Can you work these out from the model? Positions are in its coordinate system, mm. A direction names the side the tool comes from. Give positions to 0.01 mm unless a question says otherwise; leave off trailing zeros. Write each loop counter-clockwise with the first axis right and the second up, starting at its lowest first coordinate (ties: lowest second). Pieces come first, ordered by that corner, then holes. Notation, with made-up numbers: M -21.5,66 L -6.5,66 A33 cw -6.5,101 Z; hole C -4.5,-24 d9. An arc over 180 degrees is marked long. Write each question's results on one line, items separated by ' | '.
from build123d import *

# Parameters (mm, degrees)
F1_DEPTH = 117.094
F4_DEPTH = 25.4
F2_R     = 16.9643352209
F2_R_2   = 9.9441
F5_DEPTH = 65.278


with BuildPart() as f1:
    # F0 (on Front) → F1 (new body)
    with BuildSketch(Plane.XZ):
        Polygon((-76.2, 0), (0, 0), (0, 152.4), (-30.48, 152.4), (-30.48, 25.4), (-76.2, 25.4), align=None)
    extrude(amount=F1_DEPTH)

    # F3 (on face) → F4 (cut)
    with BuildSketch(Plane.XY.offset(25.4)):
        with BuildLine():
            ThreePointArc((-76.2, -83.7641331735), (-50.9828668265, -58.547), (-76.2, -33.3298668265))
            Line((-76.2, -33.3298668265), (-76.2, -83.7641331735))
        make_face()
    extrude(amount=-F4_DEPTH, mode=Mode.SUBTRACT)

    # F2 (on face) → F5 (cut)
    with BuildSketch(Plane(origin=(-30.48, 0, 0), x_dir=(0, -1, 0), z_dir=(-1, 0, 0))):
        with Locations((58.547, 126.1055916548)):
            Circle(F2_R)
        with Locations((58.547, 126.1055916548)):
            Circle(F2_R_2, mode=Mode.SUBTRACT)
        with Locations((58.547, 126.1055916548)):
            Circle(F2_R_2)
    extrude(amount=-F5_DEPTH, mode=Mode.SUBTRACT)


solid = f1.part
Item 1: I'm going to push flat-ended pins straight in: pin 1 (3 mm diameter, centred on x = -60.5, y = -99.5, fed in from +Z); pin 2 (6 mm diameter, centred on y = -44, z = 21, fed in from -X). Where does each tip first touch, or does it pass through?
Geometry says:
pin 1: stops at z = 25.4 | pin 2: stops at x = -58.09
Item 2: For faces 1 (the face through (-48, -58, 25.4)), 2 (the face through (-15, -58, 152.4)), which set-ups out of +Z, -Z, +X, -X, +Y, -Y let a thin tool reach every point of the face, with its end or its side?
Geometry says:
face 1: +Z, -X, +Y, -Y | face 2: +Z, +X, -X, +Y, -Y
Item 3: I want a section at C-C, the plane y = -93.5. Please give me the cut outline in (x, z).
Geometry says:
outline: M -76.2,0 L 0,0 L 0,152.4 L -30.48,152.4 L -30.48,25.4 L -76.2,25.4 Z
Item 4: Thinking about a two-plate mould opening in Z: for faces 3 (the face through (-76.2, -100, 13)), 4 (the face through (-15.45, -74.22, 119.61)), 5 (the face through (-39, -58, 0)), which applies, +Z half, -Z half, draft (parallel to the pull), parting line (faces both ways), or undercut?
Geometry says:
face 3: draft | face 4: undercut | face 5: -Z half
Item 5: I want a section at A-A, the plane y = -43.5. Please give me the cut outline in (x, z).
Geometry says:
outline: M -55.96,0 L 0,0 L 0,118.27 L -30.48,118.27 L -30.48,25.4 L -55.96,25.4 Z; M -30.48,133.94 L 0,133.94 L 0,152.4 L -30.48,152.4 Z
Item 6: If I drill on line 1 (X direction, y = -80, z = 85); line 2 (Z direction, x = -65, y = -93); line 3 (Y direction, x = -16, z = 114), over which ranges is the centre line in solid material (lowest first)? Write a range as from..to.
Geometry says:
line 1: x = -30.48..0 | line 2: z = 0..25.4 | line 3: y = -117.09..-70.43, -46.66..0
Item 7: I want a section at D-D, the plane z = 16. Please give me the cut outline in (x, y).
Geometry says:
outline: M -76.2,-117.09 L 0,-117.09 L 0,0 L -76.2,0 L -76.2,-33.33 A25.22 cw -76.2,-83.76 Z
Item 8: I want a section at B-B, the plane z = 113.5. Please give me the cut outline in (x, y).
Geometry says:
outline: M -30.48,-117.09 L 0,-117.09 L 0,-69.9 L -30.48,-69.9 Z; M -30.48,-47.19 L 0,-47.19 L 0,0 L -30.48,0 Z
